The figure shows three views and two pictorial views of one solid part (mm, origin at its lowest corner). Answer the questions. A direction names the side the tool comes from. Coordinates: 2 decimals unless noted, no trailing zeros. Order: outer loops, then holes, each group sorted by start corner. A loop starts at its lowest first (then second) coordinate and runs counter-clockwise, first axis right, second up.
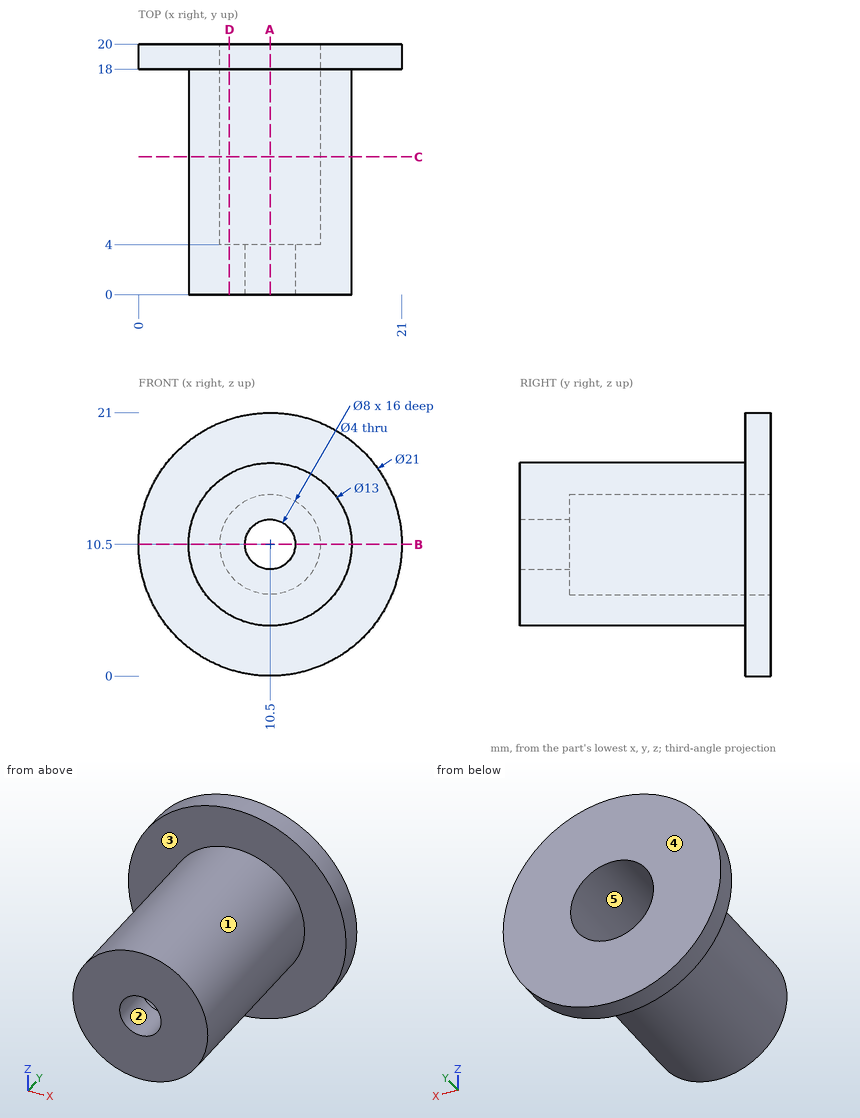
1) The mould has two halves that part along X. Classify the marked faces 1, 2 and 3: released by +X, released by -X, zero draft, split by the parting line, or undercut.
2) A cutting plane is placed at A-A, the plane x = 10.5. Write down the section's boundary in (y, z).
3) A cutting plane is placed at C-C, the plane y = 11. Write down the section's boundary in (x, z), plus the area to 3 significant figures.
4) Straight lines are drawn through the part: probe 1 along X at (y, z) = (3.1, 10.5); probe 2 along Z at (x, y) = (10.5, 7.5). For each, find the intervals that lie inside material, in ascending order.
5) Each of these flat-tipped pins is pushed along its axis until it touches: P1, Ø1, axis at y = 3, z = 13, coming from the -X side; P2, Ø6, axis at x = 7, y = 11, coming from the +Z side; P3, Ø8, axis at y = 7, z = 9, coming from the +X side. Where does it stop, or does it pass through?
6) A cutting plane is placed at D-D, the plane x = 7.25. Write down the section's boundary in (y, z).
7) For the marked faces 4 and 5, determine the directions among +Z, -Z, +X, -X, +Y, -Y from which every point of the face is accessible in a straight line to the end or side of a thin tool.
8) A cutting plane is placed at B-B, the plane z = 10.5. Write down the section's boundary in (x, y).
Working result:
1. face 1: split by the parting line
1. face 2: undercut
1. face 3: zero draft
2. outline: (0, 4) - (18, 4) - (18, 0) - (20, 0) - (20, 6.5) - (4, 6.5) - (4, 8.5) - (0, 8.5) - close; (0, 12.5) - (4, 12.5) - (4, 14.5) - (20, 14.5) - (20, 21) - (18, 21) - (18, 17) - (0, 17) - close
3. outline: circle Ø13 at (10.5, 10.5); hole circle Ø8 at (10.5, 10.5)
3. area: 82.5 mm2
4. probe 1: x = 4 to 8.5, 12.5 to 17
4. probe 2: z = 4 to 6.5, 14.5 to 17
5. P1: stops at x = 4.32
5. P2: stops at z = 16.98
5. P3: stops at x = 17
6. outline: (0, 4.87) - (18, 4.87) - (18, 0.52) - (20, 0.52) - (20, 8.17) - (4, 8.17) - (4, 12.83) - (20, 12.83) - (20, 20.48) - (18, 20.48) - (18, 16.13) - (0, 16.13) - close
7. face 4: +Z, -Z, +X, -X, +Y
7. face 5: +Y
8. outline: (0, 18) - (4, 18) - (4, 0) - (8.5, 0) - (8.5, 4) - (6.5, 4) - (6.5, 20) - (0, 20) - close; (12.5, 0) - (17, 0) - (17, 18) - (21, 18) - (21, 20) - (14.5, 20) - (14.5, 4) - (12.5, 4) - close
